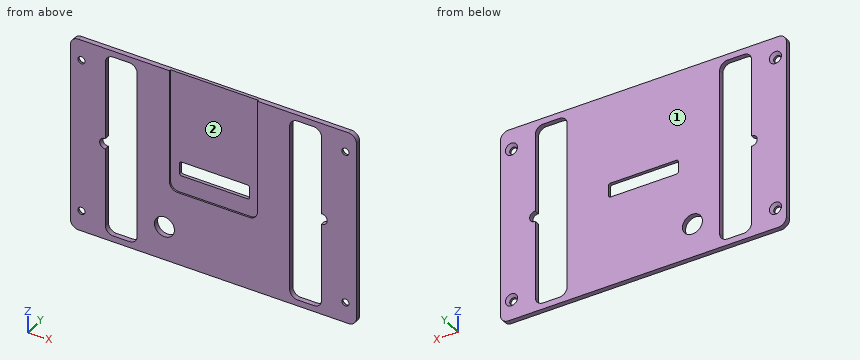
Autodesk Inventor part; units mm, degrees
ref_plane "YZ Plane" through (0, 0, 0) normal (1, 0, 0) x (0, 1, 0)
ref_plane "XZ Plane" through (0, 0, 0) normal (0, 1, 0) x (-1, 0, 0)
ref_plane "XY Plane" through (0, 0, 0) normal (0, 0, 1) x (1, 0, 0)
sketch "Sketch1" plane through (0, 0, 0) normal (0, 1, 0) x (-1, 0, 0)
  line L0 (-35.75, 24.05) -> (35.75, 24.05)
  line L1 (35.75, 24.05) -> (35.75, -24.05)
  line L2 (35.75, -24.05) -> (-35.75, -24.05)
  line L3 (-35.75, -24.05) -> (-35.75, 24.05)
  line L4 (-35.75, 24.05) -> (35.75, -24.05) construction
  line L5 (35.75, 24.05) -> (-35.75, -24.05) construction
  point P0 (0, 0)
  dimension "d0" = 48.1
  dimension "d1" = 71.5
extrude "Extrusion1" add sketch "Sketch1" along normal blind 1.23
sketch "Sketch2" plane through (0, 1.23, 0) normal (0, 1, 0) x (1, 0, 0)
  point P0 (0, 0)
  point P1 (-33, 19)
  point P2 (33, 19)
  point P3 (-33, -19)
  point P4 (33, -19)
  dimension "d77" = 38
  dimension "d78" = 19
  dimension "d79" = 33
  dimension "d115" = 33
hole "Hole1" at (-33, 1.23, -19) at (33, 1.23, -19) at (-33, 1.23, 19) at (33, 1.23, 19) direction (0, -1, 0) diameter 1.778 end through all countersink diameter 3.023 countersink angle 82
fillet "Fillet3" radius 2 4 edges at (35.75, 0.615, 24.05) (35.75, 0.615, -24.05) (-35.75, 0.615, -24.05) (-35.75, 0.615, 24.05)
sketch "Sketch10" plane through (0, 1.23, 0) normal (0, 1, 0) x (1, 0, 0)
  line L0 (-27.55, -21) -> (-29.05, -21)
  line L1 (-29.05, -21) -> (-29.05, 21)
  line L2 (-29.05, 21) -> (-27.55, 21)
  line L3 (-27.55, 21) -> (-27.55, -21)
  line L4 (-27.55, -21) -> (-29.05, 21) construction
  line L5 (-29.05, -21) -> (-27.55, 21) construction
  line L6 (0, 13.6561) -> (0, -11.4856)
  line L7 (27.55, -21) -> (29.05, -21)
  line L8 (29.05, -21) -> (29.05, 21)
  line L9 (29.05, 21) -> (27.55, 21)
  line L10 (27.55, 21) -> (27.55, -21)
  line L11 (27.55, -21) -> (29.05, 21) construction
  line L12 (29.05, -21) -> (27.55, 21) construction
  point P0 (0, 0)
  point P1 (-28.3, 0)
  point P2 (-27.55, 0)
  point P3 (28.3, 0)
  point P4 (27.55, 0)
  dimension "d124" = 1.5
  dimension "d125" = 42
  dimension "d126" = 27.55
extrude "Extrusion7" [suppressed]
sketch "Sketch11" plane through (0, 0, 0) normal (0, -1, 0) x (1, 0, 0)
  line L0 (-33.75, 24.05) -> (33.75, 24.05)
  line L1 (-11, 24.05) -> (11, 24.05)
  line L2 (11, 24.05) -> (11, -3.95)
  line L3 (9, -5.95) -> (-9, -5.95)
  line L4 (-11, -3.95) -> (-11, 24.05)
  arc A0 (9, -5.95) -> (11, -3.95) centre (9, -3.95) ccw
  arc A1 (-11, -3.95) -> (-9, -5.95) centre (-9, -3.95) ccw
  point P0 (0, 0)
  point P1 (11, -5.95)
  point P2 (-11, -5.95)
  dimension "d129" = 22
  dimension "d130" = 30
  dimension "d131" = 11
  dimension "d132" = 2
extrude "Extrusion8" cut sketch "Sketch11" against normal blind 0.43
sketch "Sketch12" plane through (0, 1.23, 0) normal (0, 1, 0) x (1, 0, 0)
  line L0 (8.25, 1.75) -> (-8.25, 1.75)
  line L1 (-8.75, 1.25) -> (-8.75, -1.25)
  line L2 (-8.25, -1.75) -> (8.25, -1.75)
  line L3 (8.75, -1.25) -> (8.75, 1.25)
  line L4 (8.75, 1.75) -> (-8.75, -1.75) construction
  line L5 (-8.75, 1.75) -> (8.75, -1.75) construction
  arc A0 (-8.75, -1.25) -> (-8.25, -1.75) centre (-8.25, -1.25) ccw
  arc A1 (-8.25, 1.75) -> (-8.75, 1.25) centre (-8.25, 1.25) ccw
  arc A2 (8.25, -1.75) -> (8.75, -1.25) centre (8.25, -1.25) ccw
  arc A3 (8.75, 1.25) -> (8.25, 1.75) centre (8.25, 1.25) ccw
  point P0 (0, 0)
  dimension "d135" = 17.5
  dimension "d136" = 3.5
  dimension "d137" = 0.5
extrude "Extrusion9" cut sketch "Sketch12" against normal through all
sketch "Sketch13" plane through (0, 1.23, 0) normal (0, 1, 0) x (1, 0, 0)
  circle A0 centre (-12.25, 15.75) radius 2.5
  point P0 (0, 0)
  dimension "d161" = 15.75
  dimension "d162" = 12.25
  dimension "d163" = 5
extrude "Extrusion10" cut sketch "Sketch13" against normal through all
sketch "Sketch15" plane through (0, 1.23, 0) normal (0, 1, 0) x (1, 0, 0)
  line L0 (-21.05, -22.55) -> (-25.05, -22.55)
  line L1 (-27.05, -20.55) -> (-27.05, 20.55)
  line L2 (-25.05, 22.55) -> (-21.05, 22.55)
  line L3 (-19.05, 20.55) -> (-19.05, -20.55)
  line L4 (-19.05, -22.55) -> (-27.05, 22.55) construction
  line L5 (-27.05, -22.55) -> (-19.05, 22.55) construction
  arc A0 (-25.05, 22.55) -> (-27.05, 20.55) centre (-25.05, 20.55) ccw
  arc A1 (-27.05, -20.55) -> (-25.05, -22.55) centre (-25.05, -20.55) ccw
  arc A2 (-21.05, -22.55) -> (-19.05, -20.55) centre (-21.05, -20.55) ccw
  arc A3 (-19.05, 20.55) -> (-21.05, 22.55) centre (-21.05, 20.55) ccw
  circle A4 centre (-27.15, 0) radius 1.3
  line L6 (0, 25.2712) -> (0, -27.2079)
  line L7 (21.05, -22.55) -> (25.05, -22.55)
  line L8 (27.05, -20.55) -> (27.05, 20.55)
  line L9 (25.05, 22.55) -> (21.05, 22.55)
  line L10 (19.05, 20.55) -> (19.05, -20.55)
  line L11 (19.05, -22.55) -> (27.05, 22.55) construction
  line L12 (27.05, -22.55) -> (19.05, 22.55) construction
  arc A5 (27.05, 20.55) -> (25.05, 22.55) centre (25.05, 20.55) ccw
  arc A6 (25.05, -22.55) -> (27.05, -20.55) centre (25.05, -20.55) ccw
  arc A7 (19.05, -20.55) -> (21.05, -22.55) centre (21.05, -20.55) ccw
  arc A8 (21.05, 22.55) -> (19.05, 20.55) centre (21.05, 20.55) ccw
  circle A9 centre (27.15, 0) radius 1.3
  point P0 (0, 0)
  point P1 (-23.05, 0)
  point P2 (-27.05, 1.2961)
  point P3 (-27.05, -1.2961)
  point P4 (23.05, 0)
  point P5 (27.05, -1.2961)
  point P6 (27.05, 1.2961)
  dimension "d164" = 45.1
  dimension "d165" = 27.05
  dimension "d166" = 2
  dimension "d167" = 8
  dimension "d170" = 27.15
  dimension "d171" = 2.6
extrude "Extrusion11" cut sketch "Sketch15" against normal through all
properties part number "spacer" material "Stainless Steel"
The model under review builds one solid part; all positions refer to its coordinate system, in mm. Face numbers are marked on the shaded views. Give positions to 0.01 mm unless a question says otherwise; leave off trailing zeros. Order: outer loops, then holes, each group sorted by start corner. A loop starts at its lowest first (then second) coordinate and runs counter-clockwise, first axis right, second up. Notation, with made-up numbers: M 75,-21 L 124,-21 A14 ccw 124,-6 Z; hole C 79.25,82.25 d9. An arc over 180 degrees is marked long. Answer in a Markdown table with one row per item. Add a question column.
1. Add section A-A on x = 33. State the section outline as (y, z) points.
2. To check wall thickness, follow line 1 along Z through (x, y) = (33, 0.25); line 2 along X through (y, z) = (0.6, -11); line 3 along X through (y, z) = (0.15, 19). State the ranges of each line that lie inside material, in increasing order.
3. Add section D-D on z = -9. State the section outline as (x, y) points, plus the area to 3 significant figures.
4. Add section C-C on x = 2. State the section outline as (y, z) points.
5. Mouldability with a two-part tool opening along X and no side actions: class the marked faces 1 and 2 as released by +X, released by -X, zero draft, split by the parting line, or undercut.
6. Add section B-B on z = 0. State the section outline as (x, y) points.
The answers:
| question | item | result |
|---|---|---|
| 1 | outline | M 0,-24.05 L 1.23,-24.05 L 1.23,-20.51 L 0.51,-19.89 L 0,-19.89 Z; M 0,-18.11 L 0.51,-18.11 L 1.23,-17.49 L 1.23,17.49 L 0.51,18.11 L 0,18.11 Z; M 0,19.89 L 0.51,19.89 L 1.23,20.51 L 1.23,24.05 L 0,24.05 Z |
| 2 | line 1 | -24.05 to -19.89, -18.11 to 18.11, 19.89 to 24.05 |
| 2 | line 2 | -35.75 to -27.05, -19.05 to 19.05, 27.05 to 35.75 |
| 2 | line 3 | -35.75 to -33.89, -32.11 to -27.05, -19.05 to -11, 11 to 19.05, 27.05 to 32.11, 33.89 to 35.75 |
| 3 | outline | M -35.75,0 L -27.05,0 L -27.05,1.23 L -35.75,1.23 Z; M -19.05,0 L 19.05,0 L 19.05,1.23 L -19.05,1.23 Z; M 27.05,0 L 35.75,0 L 35.75,1.23 L 27.05,1.23 Z |
| 3 | area | 68.3 mm2 |
| 4 | outline | M 0,-24.05 L 1.23,-24.05 L 1.23,-1.75 L 0.43,-1.75 L 0.43,-5.95 L 0,-5.95 Z; M 0.43,1.75 L 1.23,1.75 L 1.23,24.05 L 0.43,24.05 Z |
| 5 | face 1 | zero draft |
| 5 | face 2 | undercut |
| 6 | outline | M -35.75,0 L -28.45,0 L -28.45,1.23 L -35.75,1.23 Z; M -19.05,0 L -11,0 L -11,0.43 L -8.75,0.43 L -8.75,1.23 L -19.05,1.23 Z; M 8.75,0.43 L 11,0.43 L 11,0 L 19.05,0 L 19.05,1.23 L 8.75,1.23 Z; M 28.45,0 L 35.75,0 L 35.75,1.23 L 28.45,1.23 Z |
